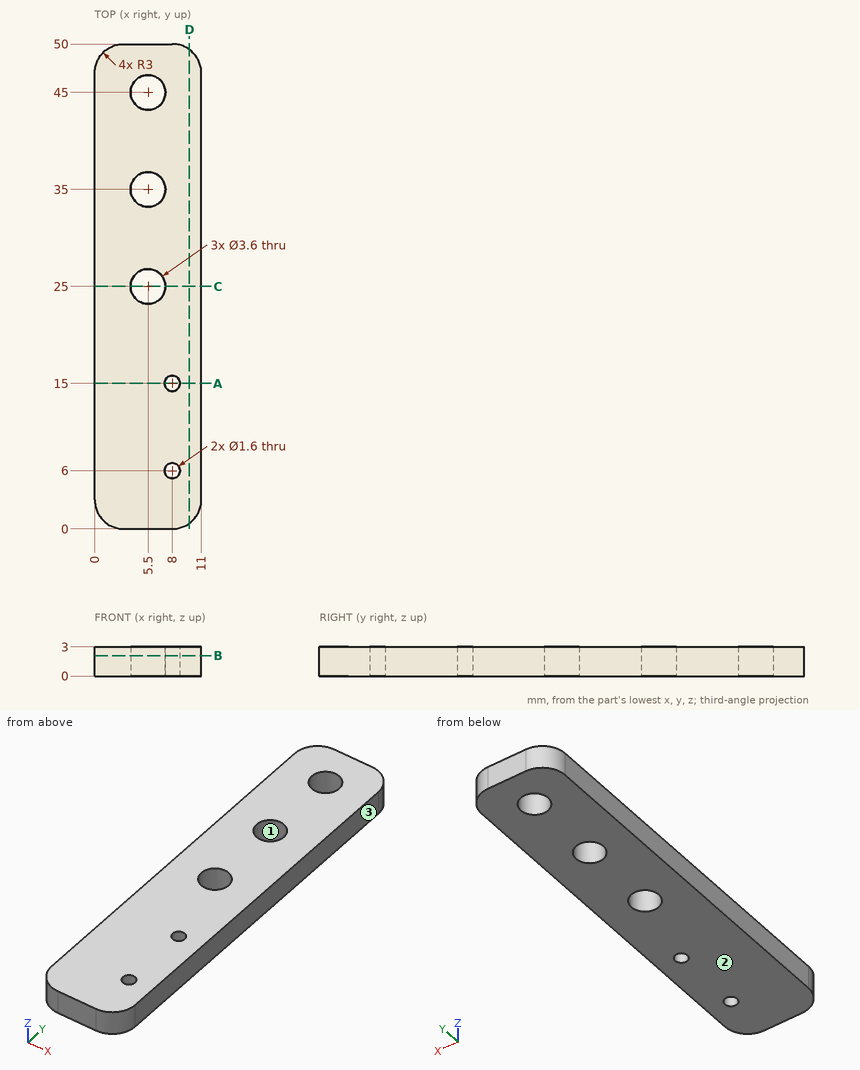
Source: three-view drawing plus pictorial views. Frame: mm from the lowest corner of the part. Round coordinates to 2 decimals unless told otherwise and drop trailing zeros. Loops run counter-clockwise (first coordinate to the right, second up) from the corner with the lowest first, then second, coordinate; pieces in that order, holes last.
Q1. Section A-A, the plane y = 15. Return loops of the section in (x, z), plus the area to 3 significant figures.
Q2. Ray query, line 1 (Y direction, x = 5.5, z = 0.9); line 2 (Y direction, x = 8, z = 2); line 3 (X direction, y = 25, z = 1.4). Return the intervals inside material, ascending.
Q3. Section C-C, the plane y = 25. Return loops of the section in (x, z), plus the area to 3 significant figures.
Q4. Section D-D, the plane x = 9.75. Return loops of the section in (y, z).
Q5. First-contact query: P1, Ø1.5, axis at x = 9, z = 0.5, coming from the +Y side. Flat tip, straight axial feed; report the tip coordinate or a pass-through.
Q6. Section B-B, the plane z = 2.1. Return loops of the section in (x, y), plus the area to 3 significant figures.
Q7. Mould query, pull axis X, two halves, no side actions, for the marked faces 1, 2 and 3. Classes: pulls with the +X half, pulls with the -X half, needs draft (parallel to the pull), parting line crosses it, or undercut.
Solutions:
1. outline: (0, 0) - (7.2, 0) - (7.2, 3) - (0, 3) - close; (8.8, 0) - (11, 0) - (11, 3) - (8.8, 3) - close
1. area: 28.2 mm2
2. line 1: y = 0 to 23.2, 26.8 to 33.2, 36.8 to 43.2, 46.8 to 50
2. line 2: y = 0 to 5.2, 6.8 to 14.2, 15.8 to 50
2. line 3: x = 0 to 3.7, 7.3 to 11
3. outline: (0, 0) - (3.7, 0) - (3.7, 3) - (0, 3) - close; (7.3, 0) - (11, 0) - (11, 3) - (7.3, 3) - close
3. area: 22.2 mm2
4. outline: (0.56, 0) - (49.44, 0) - (49.44, 3) - (0.56, 3) - close
5. P1: stops at y = 49.99
6. outline: (0, 3) arc R3 ccw to (3, 0) - (8, 0) arc R3 ccw to (11, 3) - (11, 47) arc R3 ccw to (8, 50) - (3, 50) arc R3 ccw to (0, 47) - close; hole circle Ø3.6 at (5.5, 25); hole circle Ø3.6 at (5.5, 35); hole circle Ø3.6 at (5.5, 45); hole circle Ø1.6 at (8, 6); hole circle Ø1.6 at (8, 15)
6. area: 508 mm2
7. face 1: undercut
7. face 2: needs draft
7. face 3: pulls with the +X half
